```python
from build123d import *

# Parameters (mm, degrees)
BOSS_EXTRUDE1_DEPTH = 1.5


with BuildPart() as part:
    # Sketch1 → Boss-Extrude1 (new body)
    with BuildSketch(Plane.XY):
        with BuildLine():
            Line((-66.795, -49.425), (-66.9813, 49.425))
            Line((-66.9813, 49.425), (-62.4676, 49.425))
            Line((-62.4676, 49.425), (-62.4676, 48.425))
            Line((-62.4676, 48.425), (-36.4676, 48.425))
            Line((-36.4676, 48.425), (-36.4676, 47.625))
            ThreePointArc((-36.4676, 47.625), (-32.215, 43.3724), (-27.9624, 47.625))
            Line((-27.9624, 47.625), (-27.9624, 48.425))
            Line((-27.9624, 48.425), (7.9824, 48.425))
            Line((7.9824, 48.425), (7.9824, 47.625))
            ThreePointArc((7.9824, 47.625), (8.113831006, 46.575918078), (8.5, 45.591682081))
            Line((8.5, 45.591682081), (8.5, 11.344715994))
            Line((8.5, 11.344715994), (3.5, 0.401446139))
            Line((3.5, 0.401446139), (3.5, -48.425))
            Line((3.5, -48.425), (-27.9624, -48.425))
            Line((-27.9624, -48.425), (-27.9624, -47.625))
            ThreePointArc((-27.9624, -47.625), (-32.215, -43.3724), (-36.4676, -47.625))
            Line((-36.4676, -47.625), (-36.4676, -48.425))
            Line((-36.4676, -48.425), (-62.4676, -48.425))
            Line((-62.4676, -48.425), (-62.4676, -49.425))
            Line((-62.4676, -49.425), (-66.795, -49.425))
        make_face()
    extrude(amount=BOSS_EXTRUDE1_DEPTH)


solid = part.part
```
Geometry check sheet. Reference: the model listing, model coordinates, mm. Give positions to 0.01 mm unless a question says otherwise; leave off trailing zeros. Loops run counter-clockwise (first coordinate to the right, second up) from the corner with the lowest first, then second, coordinate; pieces in that order, holes last. Notation, with made-up numbers: M 57.25,60 L 69.25,60 A12 ccw 69.25,69 Z; hole C 78.5,53.5 d6. An arc over 180 degrees is marked long. Write item = value, one per line.
(1) Sectioned sample at A-A, the plane z = 1.2. Record the cut outline in (x, y) (3 decimals), plus the area to 3 significant figures.
Answer below:
outline = M -66.981,49.425 L -66.795,-49.425 L -62.468,-49.425 L -62.468,-48.425 L -36.468,-48.425 L -36.468,-47.625 A4.253 cw -27.962,-47.625 L -27.962,-48.425 L 3.5,-48.425 L 3.5,0.401 L 8.5,11.345 L 8.5,45.592 A4.253 cw 7.982,47.625 L 7.982,48.425 L -27.962,48.425 L -27.962,47.625 A4.253 cw -36.468,47.625 L -36.468,48.425 L -62.468,48.425 L -62.468,49.425 Z
area = 6,970 mm2
(2) Sectioned sample at B-B, the plane x = -55. Record the cut outline in (y, z) (3 decimals), plus the area to 3 significant figures.
Answer below:
outline = M -48.425,0 L 48.425,0 L 48.425,1.5 L -48.425,1.5 Z
area = 145 mm2
(3) Material ranges on line 1 (Y direction, x = -18, z = 1.1) (3 decimals); line 2 (X direction, y = 45, z = 0.45); line 3 (X direction, y = -39, z = 0.4), recorded low to high. Write a range as [from, to].
Answer below:
line_1 = [-48.425, 48.425]
line_2 = [-66.97, -35.56], [-28.87, 8.5]
line_3 = [-66.81, 3.5]
(4) Gauge pin test, flat ends, axial feed: pin 1 Ø0.8 at (y, z) = (-49, 1) entering from +X; pin 2 Ø0.8 at (x, z) = (-17.5, 0.5) entering from +Y (3 decimals). Record the tip position at first contact, or that the pin passes through.
Answer below:
pin_1 = -62.47
pin_2 = 48.425
(5) Release check for a two-part mould opening along X. For faces 1 (the face through (-29, 1, 0)), 2 (the face through (6.035, 5.95, 0.74)), 3 (the face through (-32.121, -43.373, 0.74)) record: released by +X, released by -X, zero draft, split by the parting line, or undercut.
Answer below:
face_1 = zero draft
face_2 = released by +X
face_3 = undercut
(6) Sectioned sample at C-C, the plane y = -41.5. Record the cut outline in (x, z).
Answer below:
outline = M -66.81,0 L 3.5,0 L 3.5,1.5 L -66.81,1.5 Z
